Design review of the part built by this model. Coordinates are the model's own, in mm. A direction names the side the tool comes from. Coordinates: 2 decimals unless noted, no trailing zeros. Loops run counter-clockwise (first coordinate to the right, second up) from the corner with the lowest first, then second, coordinate; pieces in that order, holes last. Notation, with made-up numbers: M 16,-2.5 L 56,-2.5 A22 cw 56,11.5 Z; hole C 70.25,10 d11. An arc over 180 degrees is marked long. Put each result on its own line as item: value. Start each with the question number.
(1) For faces 1 (the cylindrical face through (-17.87, 17.77, 12.82)), 2 (the cylindrical face through (40.993, 1.911, 23.505)), 3 (the cylindrical face through (36.746, -0.179, 22.866)), list the 3-axis set-ups (+Z, -Z, +X, -X, +Y, -Y) from which the entire face can be reached by the end or side of a thin tool; tool diameter is ignored.
(2) Take a section at B-B, the plane y = 17. Give the boundary of the cut face in (x, z).
(3) For probe 1 along Y at (x, z) = (-7.5, 8.75); probe 2 along X at (y, z) = (1, 24.5); probe 3 along X at (y, z) = (-19.5, 14), list the stretches that pass through material, from the lowest coordinate up. Write a range as [from, to].
(4) Take a section at C-C, the plane z = 11.5. Give the boundary of the cut face in (x, y).
(5) Clearance check with flat-ended pins moving along their axes: pin 1 (3 mm diameter, centred on y = 11.5, z = 3.5, fed in from +X); pin 2 (3 mm diameter, centred on y = -29.5, z = 16, fed in from -X); pin 3 (12 mm diameter, centred on x = 16, z = 12.5, fed in from -Y); pin 4 (11 mm diameter, centred on y = -30.5, z = 13.5, fed in from +X). State where each tip first meets the part, or that it passes through.
(6) Take a section at A-A, the plane x = 9. Give the boundary of the cut face in (y, z).
(7) The part is to be moulded in two halves that separate along X. For faces 4 (the flat face through (-21.1, 0, 13)), 5 (the flat face through (45.1, 1, 21)), 6 (the flat face through (-14.921, -30, 13)), say which applies: +X half, -X half, draft (parallel to the pull), parting line (faces both ways), or undercut.
```python
from build123d import *

# Parameters (mm, degrees)
EXTRUDE_THIN1_DEPTH        = 26
SKETCH2_R                  = 2.5
BOSS_EXTRUDE1_DEPTH        = 20
BOSS_EXTRUDE2_START        = -50.2
SKETCH2_3_R                = 2.5
BOSS_EXTRUDE2_DEPTH        = 20
SKETCH3_W                  = 29.841581728
SKETCH3_H                  = 26
BOSS_EXTRUDE3_DEPTH        = 10
WYTNIJ_WYCI_GNI_CIE1_START = -8.6
SZKIC1_R                   = 2.5
SZKIC1_R_2                 = 2.2
WYTNIJ_WYCI_GNI_CIE1_DEPTH = 0.5
WYTNIJ_WYCI_GNI_CIE2_START = -8.6
SZKIC2_R                   = 2.5
SZKIC2_R_2                 = 2.2
WYTNIJ_WYCI_GNI_CIE2_DEPTH = 0.5


with BuildPart() as part:
    # Sketch1 → Extrude-Thin1 (new body)
    with BuildSketch(Plane.XY):
        with BuildLine():
            Line((-25.1, -14.920790864), (-25.1, 14.920790864))
            ThreePointArc((-25.1, 14.920790864), (-20.647518011, 20.647518011), (-14.920790864, 25.1))
            Line((-14.920790864, 25.1), (14.920790864, 25.1))
            ThreePointArc((14.920790864, 25.1), (20.647518011, 20.647518011), (25.1, 14.920790864))
            Line((25.1, 14.920790864), (25.1, -14.920790864))
            ThreePointArc((25.1, -14.920790864), (20.647518011, -20.647518011), (14.920790864, -25.1))
            Line((14.920790864, -25.1), (-14.920790864, -25.1))
            ThreePointArc((-14.920790864, -25.1), (-20.647518011, -20.647518011), (-25.1, -14.920790864))
        make_face()
        with BuildLine():
            Line((-21.1, -13.777880824), (-21.1, 13.777880824))
            ThreePointArc((-21.1, 13.777880824), (-17.819090886, 17.819090886), (-13.777880824, 21.1))
            Line((-13.777880824, 21.1), (13.777880824, 21.1))
            ThreePointArc((13.777880824, 21.1), (17.819090886, 17.819090886), (21.1, 13.777880824))
            Line((21.1, 13.777880824), (21.1, -13.777880824))
            ThreePointArc((21.1, -13.777880824), (17.819090886, -17.819090886), (13.777880824, -21.1))
            Line((13.777880824, -21.1), (-13.777880824, -21.1))
            ThreePointArc((-13.777880824, -21.1), (-17.819090886, -17.819090886), (-21.1, -13.777880824))
        make_face(mode=Mode.SUBTRACT)
    extrude(amount=EXTRUDE_THIN1_DEPTH)

    # Sketch2 → Boss-Extrude1 (add)
    with BuildSketch(Plane.ZY.offset(25.1)):
        with Locations((21.12, 1.16)):
            Circle(SKETCH2_R)
    extrude(amount=BOSS_EXTRUDE1_DEPTH)

    # Sketch2<3> → Boss-Extrude2 (add)
    with BuildSketch(Plane.ZY.offset(25.1).offset(BOSS_EXTRUDE2_START)):
        with Locations((21.12, 1.16)):
            Circle(SKETCH2_3_R)
    extrude(amount=-BOSS_EXTRUDE2_DEPTH)

    # Sketch3 → Boss-Extrude3 (add)
    with BuildSketch(Plane.XZ.offset(25.1)):
        with Locations((0, 13)):
            Rectangle(SKETCH3_W, SKETCH3_H)
    extrude(amount=BOSS_EXTRUDE3_DEPTH)

    # Szkic1 → Wytnij-wyciągnięcie1 (cut)
    with BuildSketch(Plane(origin=(45.1, 0, 0), x_dir=(0, 0, -1), z_dir=(1, 0, 0)).offset(WYTNIJ_WYCI_GNI_CIE1_START)):
        with Locations((-21.12, 1.16)):
            Circle(SZKIC1_R)
        with Locations((-21.12, 1.16)):
            Circle(SZKIC1_R_2, mode=Mode.SUBTRACT)
    extrude(amount=WYTNIJ_WYCI_GNI_CIE1_DEPTH, mode=Mode.SUBTRACT)

    # Szkic2 → Wytnij-wyciągnięcie2 (cut)
    with BuildSketch(Plane.ZY.offset(45.1).offset(WYTNIJ_WYCI_GNI_CIE2_START)):
        with Locations((21.12, 1.16)):
            Circle(SZKIC2_R)
        with Locations((21.12, 1.16)):
            Circle(SZKIC2_R_2, mode=Mode.SUBTRACT)
    extrude(amount=WYTNIJ_WYCI_GNI_CIE2_DEPTH, mode=Mode.SUBTRACT)


solid = part.part
```
Computed values:
1. face 1: +Z, -Z
1. face 2: +X
1. face 3: none
2. outline: M -23.74,0 L -18.6,0 L -18.6,26 L -23.74,26 Z; M 18.6,0 L 23.74,0 L 23.74,26 L 18.6,26 Z
3. probe 1: y = [-35.1, -21.1], [21.1, 25.1]
3. probe 2: x = [-25.1, -21.1], [21.1, 25.1]
3. probe 3: x = [-21.73, -15.96], [15.96, 21.73]
4. outline: M -25.1,-14.92 A29.2 ccw -14.92,-25.1 L -14.92,-35.1 L 14.92,-35.1 L 14.92,-25.1 A29.2 ccw 25.1,-14.92 L 25.1,14.92 A29.2 ccw 14.92,25.1 L -14.92,25.1 A29.2 ccw -25.1,14.92 Z; hole M -21.1,-13.78 A25.2 ccw -13.78,-21.1 L 13.78,-21.1 A25.2 ccw 21.1,-13.78 L 21.1,13.78 A25.2 ccw 13.78,21.1 L -13.78,21.1 A25.2 ccw -21.1,13.78 Z
5. pin 1: stops at x = 25.1
5. pin 2: stops at x = -14.92
5. pin 3: stops at y = -35.1
5. pin 4: stops at x = 15.09
6. outline: M -35.1,0 L -21.1,0 L -21.1,26 L -35.1,26 Z; M 21.1,0 L 25.1,0 L 25.1,26 L 21.1,26 Z
7. face 4: undercut
7. face 5: +X half
7. face 6: -X half
